```python
from build123d import *

# Parameters (mm, degrees)
F0_W      = 59
F0_H      = 51.5
F1_DEPTH  = 26.8
F2_W      = 10
F2_H      = 13
F3_DEPTH  = 26.8
F4_W      = 12.999998
F4_H      = 13
F5_DEPTH  = 22.75
F7_DEPTH  = 51.5
F9_DEPTH  = 51.5
F10_W     = 10
F10_H     = 8.67
F11_DEPTH = 38.5
F12_W     = 13
F12_H     = 3
F13_DEPTH = 5


with BuildPart() as f1:
    # F0 (on Top) → F1 (new body)
    with BuildSketch(Plane.XY):
        Rectangle(F0_W, F0_H)
    extrude(amount=F1_DEPTH)

    # F2 (on face) → F3 (cut)
    with BuildSketch(Plane.XY.offset(26.8)):
        with Locations((0, -19.25)):
            Rectangle(F2_W, F2_H)
    extrude(amount=-F3_DEPTH, mode=Mode.SUBTRACT)

    # F4 (on face) → F5 (cut)
    with BuildSketch(Plane.XY.offset(26.8)):
        with Locations((-1e-06, -19.25)):
            Rectangle(F4_W, F4_H)
    extrude(amount=-F5_DEPTH, mode=Mode.SUBTRACT)

    # F6 (on face) → F7 (cut)
    with BuildSketch(Plane.XZ.offset(25.75)):
        Polygon((-29.5, 26.8), (-29.5, 0), (-10.244871, 26.8), align=None)
    extrude(amount=-F7_DEPTH, mode=Mode.SUBTRACT)

    # F8 (on face) → F9 (cut)
    with BuildSketch(Plane.XZ.offset(25.75)):
        Polygon((10.244871, 26.8), (29.5, 0), (29.5, 26.8), align=None)
    extrude(amount=-F9_DEPTH, mode=Mode.SUBTRACT)

    # F10 (on face) → F11 (cut)
    with BuildSketch(Plane.XZ.offset(12.75)):
        with Locations((0, 4.302397)):
            Rectangle(F10_W, F10_H)
    extrude(amount=-F11_DEPTH, mode=Mode.SUBTRACT)

    # F12 (on face) → F13 (cut)
    with BuildSketch(Plane.XZ.offset(12.75)):
        with Locations((0, 23.3)):
            Rectangle(F12_W, F12_H)
    extrude(amount=-F13_DEPTH, mode=Mode.SUBTRACT)


solid = f1.part
```
Verification items for the finished model (mm, model axes). A direction names the side the tool comes from. Coordinates: 2 decimals unless noted, no trailing zeros. Loops run counter-clockwise (first coordinate to the right, second up) from the corner with the lowest first, then second, coordinate; pieces in that order, holes last. Notation, with made-up numbers: (65.5, 21.5) -> (123.5, 21.5) arc R19 ccw to (123.5, 43.5) -> close; hole circle Ø5 at (88.25, 10.5). An arc over 180 degrees is marked (long way). Answer in a Markdown table with one row per item.
1) Section check D-D (z = 7.5). Record the cut outline in (x, y).
The answers:
| item | result |
|---|---|
| outline | (-24.11, -25.75) -> (-6.5, -25.75) -> (-6.5, -12.75) -> (-5, -12.75) -> (-5, 25.75) -> (-24.11, 25.75) -> close; (5, -12.75) -> (6.5, -12.75) -> (6.5, -25.75) -> (24.11, -25.75) -> (24.11, 25.75) -> (5, 25.75) -> close |
2) Access from +Z, -Z, +X, -X, +Y, -Y to the whole of each face (thin tool, end or side, straight path). Record for faces 1 (the face through (0, -12.75, 26)), 2 (the face through (0, -10, 21.8)), 3 (the face through (5, 0, 4)).
The answers:
| item | result |
|---|---|
| face 1 | +Z, -Y |
| face 2 | -Y |
| face 3 | -Z, +Y, -Y |
3) Section check C-C (x = 4). Record the cut outline in (y, z).
The answers:
| item | result |
|---|---|
| outline | (-12.75, 8.64) -> (25.75, 8.64) -> (25.75, 26.8) -> (-12.75, 26.8) -> (-12.75, 24.8) -> (-7.75, 24.8) -> (-7.75, 21.8) -> (-12.75, 21.8) -> close |
4) Scan lines: line 1 along Z through (x, y) = (3, -9.5); line 2 along X through (y, z) = (-12, 24); line 3 along Z through (x, y) = (3.5, 17.5). Record each from-to range of solid material in increasing order. Write a range as from..to.
The answers:
| item | result |
|---|---|
| line 1 | z = 8.64..21.8, 24.8..26.8 |
| line 2 | x = -12.26..-6.5, 6.5..12.26 |
| line 3 | z = 8.64..26.8 |
5) Depth check by flat-ended pin: P1, Ø1.5, axis at y = 1.5, z = 10.5, coming from the +X side; P2, Ø7, axis at y = -4.5, z = 2.5, coming from the -X side; P3, Ø10.5, axis at y = -19.5, z = 11, coming from the -X side; P4, Ø1.5, axis at x = 17.5, z = 18.5, coming from the -Y side. Enter the tip coordinate at first touch or a pass-through.
The answers:
| item | result |
|---|---|
| P1 | stops at x = 22.49 |
| P2 | stops at x = -29.5 |
| P3 | stops at x = -25.37 |
| P4 | passes through |
6) Draft check along X on faces 4 (the face through (-5, 0, 4)), 5 (the face through (-6.5, -19, 16)), 6 (the face through (0, 25.75, 10)), 7 (the face through (-20.01, -0.36, 13.21)). Enter one of: released by +X, released by -X, zero draft, split by the parting line, or undercut.
The answers:
| item | result |
|---|---|
| face 4 | undercut |
| face 5 | undercut |
| face 6 | zero draft |
| face 7 | released by -X |
7) Section check A-A (y = -15.5). Record the cut outline in (x, z), and give its area (3 significant figures).
The answers:
| item | result |
|---|---|
| outline | (-29.5, 0) -> (-5, 0) -> (-5, 4.05) -> (-6.5, 4.05) -> (-6.5, 26.8) -> (-10.24, 26.8) -> close; (5, 0) -> (29.5, 0) -> (10.24, 26.8) -> (6.5, 26.8) -> (6.5, 4.05) -> (5, 4.05) -> close |
| area | 729 mm2 |
8) Section check B-B (y = -5). Record the cut outline in (x, z).
The answers:
| item | result |
|---|---|
| outline | (-29.5, 0) -> (-5, 0) -> (-5, 8.64) -> (5, 8.64) -> (5, 0) -> (29.5, 0) -> (10.24, 26.8) -> (-10.24, 26.8) -> close |
